Check sheet for the modelled part. Datum: model origin and axes. Units: mm. Face numbers are marked on the shaded views. A direction names the side the tool comes from. Round coordinates to 2 decimals unless told otherwise and drop trailing zeros. Order: outer loops, then holes, each group sorted by start corner. A loop starts at its lowest first (then second) coordinate and runs counter-clockwise, first axis right, second up. Notation, with made-up numbers: (30, 19.5) -> (73, 19.5) arc R21 cw to (73, 40.5) -> close; hole circle Ø7 at (83, -5.75). An arc over 180 degrees is marked (long way). Answer in a Markdown table with one row per item.
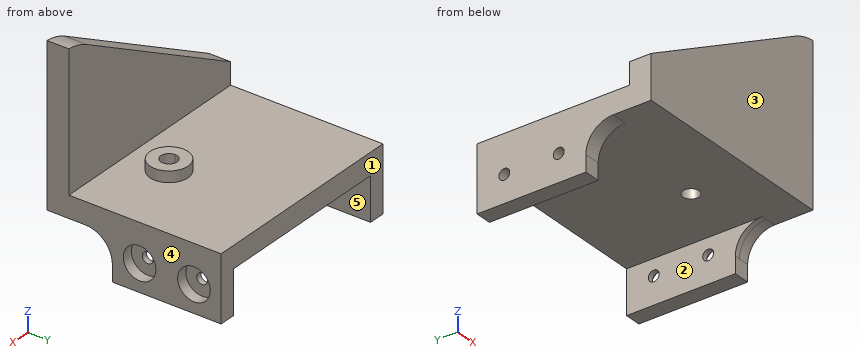
from build123d import *

# Parameters (mm, degrees)
BOSS_EXTRUDE1_DEPTH     = 20
SKETCH2_W               = 37.5
SKETCH2_H               = 4
BOSS_EXTRUDE2_DEPTH     = 12
FILLET1_R               = 5
SKETCH3_W               = 37.5
SKETCH3_H               = 4
BOSS_EXTRUDE3_DEPTH     = 25
SKETCH4_R               = 3.5
SKETCH4_R_2             = 1.5
BOSS_EXTRUDE4_DEPTH     = 2
SKETCH5_R               = 1.5
CUT_EXTRUDE1_DEPTH      = 49.324424466
CUT_EXTRUDE2_DEPTH      = 10
CUT_EXTRUDE3_DEPTH      = 50.307707308
CUT_EXTRUDE3_DEPTH_BACK = 50.307707308
SKETCH8_R               = 1
SKETCH9_R               = 3
BOSS_EXTRUDE5_DEPTH     = 2
FILLET2_R               = 10


with BuildPart() as part:
    # Sketch1 → Boss-Extrude1 (new body)
    with BuildSketch(Plane(origin=(0, 0, 0), x_dir=(1, 0, 0), z_dir=(0, 1, 0))):
        Polygon((0, 12), (0, 0), (37.5, 0), (37.5, 12), (36.5, 12), (36.5, 4), (3, 4), (3, 12), align=None)
    extrude(amount=BOSS_EXTRUDE1_DEPTH)

    # Sketch2 → Boss-Extrude2 (add)
    with BuildSketch(Plane.XZ):
        with Locations((18.75, -2)):
            Rectangle(SKETCH2_W, SKETCH2_H)
    extrude(amount=BOSS_EXTRUDE2_DEPTH)

    # Fillet1
    fillet1_edges = [part.edges().sort_by_distance(p)[0] for p in [
        (37, 0, -4),
        (1.5, 0, -4),
    ]]
    fillet(fillet1_edges, radius=FILLET1_R)

    # Sketch3 → Boss-Extrude3 (add)
    with BuildSketch(Plane.XY):
        with Locations((18.75, -10)):
            Rectangle(SKETCH3_W, SKETCH3_H)
    extrude(amount=BOSS_EXTRUDE3_DEPTH)

    # Sketch4 → Boss-Extrude4 (add)
    with BuildSketch(Plane.XY):
        with Locations(Location((25, -0.5, 0), (0, 0, 180))):
            Circle(SKETCH4_R)
        with Locations((25, -0.5)):
            Circle(SKETCH4_R_2, mode=Mode.SUBTRACT)
    extrude(amount=BOSS_EXTRUDE4_DEPTH)

    # Sketch5 → Cut-Extrude1 (cut, through all)
    with BuildSketch(Plane.XY.offset(2)):
        with Locations(Location((25, -0.5, 0), (0, 0, 180))):
            Circle(SKETCH5_R)
    extrude(amount=-CUT_EXTRUDE1_DEPTH, mode=Mode.SUBTRACT)

    # Sketch6 → Cut-Extrude2 (cut)
    with BuildSketch(Plane(origin=(0, -8, 0), x_dir=(1, 0, 0), z_dir=(0, 1, 0))):
        Polygon((37.5, -25), (0, -4), (0, -25), align=None)
    extrude(amount=-CUT_EXTRUDE2_DEPTH, mode=Mode.SUBTRACT)

    # Sketch8 → Cut-Extrude3 (cut, two sides: drawn at the far end of the back side and taken through both)
    with BuildSketch(Plane(origin=(37.5, 0, 0), x_dir=(0, 0, -1), z_dir=(1, 0, 0)).offset(-CUT_EXTRUDE3_DEPTH_BACK)):
        with Locations((7, 15)):
            Circle(SKETCH8_R)
        with Locations((7, 5)):
            Circle(SKETCH8_R)
    extrude(amount=CUT_EXTRUDE3_DEPTH + CUT_EXTRUDE3_DEPTH_BACK, mode=Mode.SUBTRACT)

    # Sketch9 → Boss-Extrude5 (add)
    with BuildSketch(Plane(origin=(37.5, 0, 0), x_dir=(0, 0, -1), z_dir=(1, 0, 0))):
        with BuildLine():
            Line((12, 20), (0, 20))
            Line((0, 20), (0, -8))
            Line((0, -8), (-25, -8))
            Line((-25, -8), (-25, -12))
            Line((-25, -12), (4, -12))
            Line((4, -12), (4, -5))
            ThreePointArc((4, -5), (5.464466094, -1.464466094), (9, 0))
            Line((9, 0), (12, 0))
            Line((12, 0), (12, 20))
        make_face()
        with Locations(Location((7, 5, 0), (0, 0, 180))):
            Circle(SKETCH9_R, mode=Mode.SUBTRACT)
        with Locations(Location((7, 15, 0), (0, 0, 180))):
            Circle(SKETCH9_R, mode=Mode.SUBTRACT)
    extrude(amount=BOSS_EXTRUDE5_DEPTH)

    # Fillet2
    # the kernel refuses this fillet: 10 mm, written as the material it takes off along each edge
    with BuildSketch(Plane(origin=(37.5, -18.416269062, 25), x_dir=(1, 0, 0), z_dir=(0, 1, 0))) as fillet2_piece_1:
        with BuildLine():
            CenterArc((2.646740347, 9.979064431), FILLET2_R, 240.751173663, 25.540689012)
            Line((-2.239293342, 1.254004272), (-2.337014016, 1.079503069))
            Line((-2.337014016, 1.079503069), (-0.097720674, -0.174501203))
            Line((-0.097720674, -0.174501203), (0, -0.2))
            ThreePointArc((0, -0.2), (1, -0.2), (1.987065193, -0.199581289))
            Line((1.987065193, -0.199581289), (2, 0))
        make_face()
    extrude(amount=16.832538123, mode=Mode.SUBTRACT)


solid = part.part
Item 1: Cross-section at A-A (y = 15). Record the boundary of the cut face in (x, z).
Result sheet:
| item | result |
|---|---|
| outline | (0, -12) -> (3, -12) -> (3, -8) -> (0, -8) -> close; (0, -6) -> (3, -6) -> (3, -4) -> (36.5, -4) -> (36.5, -6) -> (37.5, -6) -> (37.5, -4) -> (39.5, -4) -> (39.5, 0) -> (0, 0) -> close; (36.5, -12) -> (39.5, -12) -> (39.5, -10) -> (37.5, -10) -> (37.5, -8) -> (36.5, -8) -> close |
Item 2: Depth check by flat-ended pin: P1, Ø2.5, axis at y = 5, z = -7, coming from the +X side; P2, Ø1.5, axis at y = 12, z = 2.5, coming from the +X side; P3, Ø8, axis at y = 5, z = -7, coming from the +X side; P4, Ø1, axis at x = 24, y = 5, coming from the +Z side. Enter the tip coordinate at first touch or a pass-through.
Result sheet:
| item | result |
|---|---|
| P1 | stops at x = 37.5 |
| P2 | passes through |
| P3 | stops at x = 39.5 |
| P4 | stops at z = 0 |
Item 3: Cross-section at B-B (x = 25). Record the boundary of the cut face in (y, z), and give its area (3 significant figures).
Result sheet:
| item | result |
|---|---|
| outline | (-12, -4) -> (-2, -4) -> (-2, 2) -> (-4, 2) -> (-4, 0) -> (-8, 0) -> (-8, 18) -> (-12, 18) -> close; (1, -4) -> (20, -4) -> (20, 0) -> (3, 0) -> (3, 2) -> (1, 2) -> close |
| area | 196 mm^2 |
Item 4: Cross-section at C-C (z = -7). State how many separate pieces and enclosed holes the cut face has, and give its area (3 significant figures).
Result sheet:
| item | result |
|---|---|
| separate pieces | 6 |
| enclosed holes | 0 |
| area | 82.5 mm^2 |
Item 5: Set-up check for the marked faces 1 and 2: record each of +Z, -Z, +X, -X, +Y, -Y from which the full face is reachable in a straight line by a thin tool's end or side.
Result sheet:
| item | result |
|---|---|
| face 1 | +Z, -Z, +X, -X, +Y |
| face 2 | -Z, +Y, -Y |
Item 6: Mould release check, pull along X, two halves, no side actions. Record for the marked faces 3, 4 and 5: pulls with the +X half, pulls with the -X half, needs draft (parallel to the pull), parting line crosses it, or undercut.
Result sheet:
| item | result |
|---|---|
| face 3 | needs draft |
| face 4 | pulls with the +X half |
| face 5 | undercut |
Item 7: Cross-section at D-D (x = 13.5). Record the boundary of the cut face in (y, z).
Result sheet:
| item | result |
|---|---|
| outline | (-12, -4) -> (20, -4) -> (20, 0) -> (-8, 0) -> (-8, 11.56) -> (-12, 11.56) -> close |
Item 8: Scan lines: line 1 (X direction, y = 0.5, z = -10); line 2 (X direction, y = 14, z = -8.5); line 3 (Z direction, x = 37.25, y = 5). Record each from-to range of solid material in increasing order. Write a range as [from, to].
Result sheet:
| item | result |
|---|---|
| line 1 | x = [0, 3], [36.5, 39.5] |
| line 2 | x = [0, 3], [36.5, 37.5] |
| line 3 | z = [-12, -8], [-6, 0] |
